Verification items for the finished model (mm, model axes). A direction names the side the tool comes from. Give positions to 0.01 mm unless a question says otherwise; leave off trailing zeros. Put each result on its own line as item: value. Start each with the question number.
```python
from build123d import *

# Parameters (mm, degrees)
SKETCH1_R           = 66.548
BOSS_EXTRUDE1_DEPTH = 4.572
BOSS_EXTRUDE2_START = -7.62
SKETCH2_R           = 10.16
BOSS_EXTRUDE2_DEPTH = 7.62
SKETCH3_R           = 1.6764
CUT_EXTRUDE1_DEPTH  = 7.62
CUT_EXTRUDE2_DEPTH  = 6.35
SKETCH6_R           = 1.905


with BuildPart() as part:
    # Sketch1 → Boss-Extrude1 (new body)
    with BuildSketch(Plane(origin=(0, 0, 0), x_dir=(1, 0, 0), z_dir=(0, 1, 0))):
        with Locations(Location((0, 0, 0), (0, 0, 270))):
            Circle(SKETCH1_R)
        with BuildLine():
            Line((7.937268245, 6.342347578), (22.249217727, 14.605355465))
            ThreePointArc((22.249217727, 14.605355465), (23.432669326, 16.147659616), (23.178922253, 18.07505999))
            Line((23.178922253, 18.07505999), (2.199704526, 54.412130997))
            ThreePointArc((2.199704526, 54.412130997), (0, 55.682130997), (-2.199704526, 54.412130997))
            Line((-2.199704526, 54.412130997), (-23.178922253, 18.07505999))
            ThreePointArc((-23.178922253, 18.07505999), (-23.432669326, 16.147659616), (-22.249217727, 14.605355465))
            Line((-22.249217727, 14.605355465), (-7.937268245, 6.342347578))
            ThreePointArc((-7.937268245, 6.342347578), (-8.798818102, 5.08), (-9.461268245, 3.702702148))
            Line((-9.461268245, 3.702702148), (-23.773217727, 11.965710034))
            ThreePointArc((-23.773217727, 11.965710034), (-25.700618102, 12.219457107), (-27.242922253, 11.036005508))
            Line((-27.242922253, 11.036005508), (-48.22213998, -25.301065498))
            ThreePointArc((-48.22213998, -25.301065498), (-48.22213998, -27.841065498), (-46.022435454, -29.111065498))
            Line((-46.022435454, -29.111065498), (-1.524, -29.111065498))
            Line((-1.524, -29.111065498), (-1.524, -10.045049726))
            ThreePointArc((-1.524, -10.045049726), (0, -10.16), (1.524, -10.045049726))
            Line((1.524, -10.045049726), (1.524, -29.111065498))
            Line((1.524, -29.111065498), (46.022435454, -29.111065498))
            ThreePointArc((46.022435454, -29.111065498), (48.22213998, -27.841065498), (48.22213998, -25.301065498))
            Line((48.22213998, -25.301065498), (27.242922253, 11.036005508))
            ThreePointArc((27.242922253, 11.036005508), (25.700618102, 12.219457107), (23.773217727, 11.965710034))
            Line((23.773217727, 11.965710034), (9.461268245, 3.702702148))
            ThreePointArc((9.461268245, 3.702702148), (8.798818102, 5.08), (7.937268245, 6.342347578))
        make_face(mode=Mode.SUBTRACT)
        with BuildLine():
            Line((-6.076302105, 53.793667028), (-49.624833262, -21.63460153))
            ThreePointArc((-49.624833262, -21.63460153), (-52.01382357, -22.897538736), (-54.188569544, -21.293554624))
            ThreePointArc((-54.188569544, -21.293554624), (-50.421844506, 29.111065498), (-8.653525531, 57.575455132))
            ThreePointArc((-8.653525531, 57.575455132), (-6.177061556, 56.494061928), (-6.076302105, 53.793667028))
        make_face(mode=Mode.SUBTRACT)
        with BuildLine():
            Line((-43.548531156, -32.159065498), (43.548531156, -32.159065498))
            ThreePointArc((43.548531156, -32.159065498), (45.836762015, -33.596523192), (45.535044013, -36.281900508))
            ThreePointArc((45.535044013, -36.281900508), (0, -58.222130997), (-45.535044013, -36.281900508))
            ThreePointArc((-45.535044013, -36.281900508), (-45.836762015, -33.596523192), (-43.548531156, -32.159065498))
        make_face(mode=Mode.SUBTRACT)
        with BuildLine():
            Line((49.624833262, -21.63460153), (6.076302105, 53.793667028))
            ThreePointArc((6.076302105, 53.793667028), (6.177061556, 56.494061928), (8.653525531, 57.575455132))
            ThreePointArc((8.653525531, 57.575455132), (50.421844506, 29.111065498), (54.188569544, -21.293554624))
            ThreePointArc((54.188569544, -21.293554624), (52.01382357, -22.897538736), (49.624833262, -21.63460153))
        make_face(mode=Mode.SUBTRACT)
    extrude(amount=BOSS_EXTRUDE1_DEPTH)

    # Sketch2 → Boss-Extrude2 (add)
    with BuildSketch(Plane(origin=(0, 4.572, 0), x_dir=(1, 0, 0), z_dir=(0, 1, 0)).offset(BOSS_EXTRUDE2_START)):
        with Locations(Location((0, 0, 0), (0, 0, 270))):
            Circle(SKETCH2_R)
    extrude(amount=BOSS_EXTRUDE2_DEPTH)

    # Sketch3 → Cut-Extrude1 (cut)
    with BuildSketch(Plane(origin=(0, 4.572, 0), x_dir=(1, 0, 0), z_dir=(0, 1, 0))):
        with Locations(Location((0, 0, 0), (0, 0, 270))):
            Circle(SKETCH3_R)
    extrude(amount=-CUT_EXTRUDE1_DEPTH, mode=Mode.SUBTRACT)

    # Sketch4 → Cut-Extrude2 (cut)
    with BuildSketch(Plane.XZ.offset(3.048)):
        Polygon((0, 6.858), (-5.939202219, 3.429), (-5.939202219, -3.429), (0, -6.858), (5.939202219, -3.429), (5.939202219, 3.429), align=None)
    extrude(amount=-CUT_EXTRUDE2_DEPTH, mode=Mode.SUBTRACT)

    # Sketch6 → Cut-Revolve1 (revolve, cut)
    with BuildSketch(Plane(origin=(0, 0, 0), x_dir=(0, 0, -1), z_dir=(1, 0, 0)), mode=Mode.PRIVATE) as cut_revolve1_sk:
        with Locations((66.548, 2.286)):
            Circle(SKETCH6_R)
    revolve(cut_revolve1_sk.sketch.rotate(Axis((0, 8.629088399, 0), (0, -1, 0)), 180), axis=Axis((0, 8.629088399, 0), (0, -1, 0)), mode=Mode.SUBTRACT)


solid = part.part
```
1) Depth check by flat-ended pin: P1, Ø2.5, axis at y = 2, z = 18, coming from the -X side; P2, Ø3.5, axis at x = 6, y = 2.5, coming from the +Z side; P3, Ø3.5, axis at x = 14.5, y = 3, coming from the -Z side. Enter the tip coordinate at first touch or a pass-through.
2) Draft check along Z on faces 1 (the face through (-4, -3.048, -5)), 2 (the face through (-1, 2, 32.159)), 3 (the face through (65.982, 0.188, -8.663)). Enter one of: pulls with the +Z half, pulls with the -Z half, needs draft (parallel to the pull), parting line crosses it, or undercut.
3) Scan lines: line 1 along X through (y, z) = (4, -29.5); line 2 along Z through (x, y) = (21, 1.75); line 3 along X through (y, z) = (0.75, -17). Record each from-to range of solid material in increasing order. Write a range as from..to.
4) Section check A-A, the plane z = 0. State how many separate pieces and enclosed holes the cut face has, plus the area to 3 significant figures.
5) Set-up check for faces 4 (the face through (0.732, 2.254, 58.218)), 5 (the face through (-5.939, 0, 0)): record each of +Z, -Z, +X, -X, +Y, -Y from which the full face is reachable in a straight line by a thin tool's end or side.
Results are:
1. P1: stops at x = -62.93
1. P2: stops at z = 66.32
1. P3: stops at z = -65.22
2. face 1: needs draft
2. face 2: undercut
2. face 3: parting line crosses it
3. line 1: x = -58.72..-50.2, -20.1..-16.58, 16.58..20.1, 50.2..58.72
3. line 2: z = -61.22..-54.3, -27.95..-21.85, -13.88..-10.36, 29.11..32.16, 54.3..61.22
3. line 3: x = -63.17..-55.68, -27.32..-23.51, 23.51..27.32, 55.68..63.17
4. separate pieces: 6
4. enclosed holes: 0
4. area: 172 mm2
5. face 4: +Y, -Y
5. face 5: -Y
